Check sheet for the modelled part. Datum: model origin and axes. Units: mm. A direction names the side the tool comes from. Round coordinates to 2 decimals unless told otherwise and drop trailing zeros. Write each loop counter-clockwise with the first axis right and the second up, starting at its lowest first coordinate (ties: lowest second). Pieces come first, ordered by that corner, then holes. Notation, with made-up numbers: (54.5, 56) - (60.5, 56) arc R26 ccw to (60.5, 78) - close; hole circle Ø5 at (84.25, 18). An arc over 180 degrees is marked (long way). Use one line per item in the form item = value. Start each with the question number.
1) Section check A-A (y = 10.5). Record the boundary of the cut face in (x, z) (3 decimals), then the cut area to 3 significant figures.
2) Section check C-C (y = -17.8). Record the boundary of the cut face in (x, z) (3 decimals).
3) Section check B-B (x = 5.75). Record the boundary of the cut face in (y, z) (3 decimals).
4) Section check D-D (x = 11). Record the boundary of the cut face in (y, z).
5) Draft check along X on faces 5 (the face through (-2.93, -17.835, -0.555)), 6 (the face through (3.5, -17.8, -1.6)), 7 (the face through (0, -13.3, -1)), 8 (the face through (12.7, 0, 1)). Enter one of: +X half, -X half, draft (parallel to the pull), parting line (faces both ways), or undercut.
6) Set-up check for faces 1 (the face through (4.301, -16.751, -0.285)), 2 (the face through (-8.2, 16, -1)), 3 (the face through (10.2, 16, -1)), 4 (the face through (8, -18, -2)): record each of +Z, -Z, +X, -X, +Y, -Y from which the full face is reachable in a straight line by a thin tool's end or side.
7) Gauge pin test, flat ends, axial feed: P1, Ø1.6, axis at y = 6.5, z = 3, coming from the +X side (3 decimals); P2, Ø2, axis at x = -9, y = 16, coming from the -Z side; P3, Ø0.5, axis at y = -17.5, z = -1.5, coming from the -X side. Record the tip position at first contact, or that the pin passes through.
8) Scan lines: probe 1 along Y at (x, z) = (0.25, -2); probe 2 along X at (y, z) = (-17, -0.5) (3 decimals); probe 3 along Y at (x, z) = (4, 2) (3 decimals). Record each from-to range of solid material in increasing order.
from build123d import *

# Parameters (mm, degrees)
SKETCH1_W           = 25.4
SKETCH1_H           = 40.6
BOSS_EXTRUDE1_DEPTH = 1.7
SKETCH2_W           = 8
SKETCH2_H           = 7
BOSS_EXTRUDE2_DEPTH = 2.5
CUT_EXTRUDE2_DEPTH  = 5
FILLET1_R           = 1
FILLET2_R           = 1
SKETCH4_W           = 18.8
SKETCH4_H           = 19.2
BOSS_EXTRUDE3_DEPTH = 2.5
SKETCH5_R           = 1.75
BOSS_EXTRUDE4_DEPTH = 2
SKETCH6_W           = 0.5
SKETCH6_H           = 1
BOSS_EXTRUDE5_DEPTH = 0.5
SKETCH7_W           = 2
SKETCH7_H           = 3
BOSS_EXTRUDE6_DEPTH = 2
SKETCH8_W           = 15.875
SKETCH8_H           = 15.875
SKETCH8_H_2         = 19.05
BOSS_EXTRUDE7_DEPTH = 2


with BuildPart() as part:
    # Sketch1 → Boss-Extrude1 (new body)
    with BuildSketch(Plane.XY):
        Rectangle(SKETCH1_W, SKETCH1_H)
    extrude(amount=BOSS_EXTRUDE1_DEPTH)

    # Sketch2 → Boss-Extrude2 (add)
    with BuildSketch(Plane.XY):
        with Locations((0, -16.8)):
            Rectangle(SKETCH2_W, SKETCH2_H)
    extrude(amount=-BOSS_EXTRUDE2_DEPTH)

    # Sketch3 → Cut-Extrude2 (cut)
    with BuildSketch(Plane.XZ.offset(20.3)):
        Polygon((3.5, -2.125), (3.5, -1.125), (2.375, 0), (-2.375, 0), (-3.5, -1.125), (-3.5, -2.125), align=None)
    extrude(amount=-CUT_EXTRUDE2_DEPTH, mode=Mode.SUBTRACT)

    # Fillet1
    fillet1_edges = [part.edges().sort_by_distance(p)[0] for p in [
        (4, -16.8, -2.5),
        (-4, -16.8, -2.5),
    ]]
    fillet(fillet1_edges, radius=FILLET1_R)

    # Fillet2
    fillet2_edges = [part.edges().sort_by_distance(p)[0] for p in [
        (4, -16.8, 0),
        (-4, -16.8, 0),
    ]]
    fillet(fillet2_edges, radius=FILLET2_R)

    # Sketch4 → Boss-Extrude3 (add)
    with BuildSketch(Plane(origin=(0, 0, 0), x_dir=(-1, 0, 0), z_dir=(0, 0, -1))):
        Rectangle(SKETCH4_W, SKETCH4_H)
    extrude(amount=BOSS_EXTRUDE3_DEPTH)

    # Sketch5 → Boss-Extrude4 (add)
    with BuildSketch(Plane(origin=(0, 0, 0), x_dir=(-1, 0, 0), z_dir=(0, 0, -1))):
        with Locations((-8.2, -17.8)):
            Circle(SKETCH5_R)
    extrude(amount=BOSS_EXTRUDE4_DEPTH)

    # Sketch6 → Boss-Extrude5 (add)
    with BuildSketch(Plane(origin=(0, 0, 0), x_dir=(-1, 0, 0), z_dir=(0, 0, -1))):
        with Locations((-7.2, -11.1)):
            Rectangle(SKETCH6_W, SKETCH6_H)
        with Locations((-6.45, -11.1)):
            Rectangle(SKETCH6_W, SKETCH6_H)
    extrude(amount=BOSS_EXTRUDE5_DEPTH)

    # Sketch7 → Boss-Extrude6 (add)
    with BuildSketch(Plane(origin=(0, 0, 0), x_dir=(-1, 0, 0), z_dir=(0, 0, -1))):
        with Locations((-9.2, 16.3)):
            Rectangle(SKETCH7_W, SKETCH7_H)
        with Locations((9.2, 16.3)):
            Rectangle(SKETCH7_W, SKETCH7_H)
    extrude(amount=BOSS_EXTRUDE6_DEPTH)

    # Sketch8 → Boss-Extrude7 (add)
    with BuildSketch(Plane.XY.offset(1.7)):
        with Locations((-1.7625, 9.8625)):
            Rectangle(SKETCH8_W, SKETCH8_H)
        with Locations((0.2375, -9.6)):
            Rectangle(SKETCH8_W, SKETCH8_H_2)
    extrude(amount=BOSS_EXTRUDE7_DEPTH)


solid = part.part
Results are:
q1.outline = (-12.7, 0) - (12.7, 0) - (12.7, 1.7) - (6.175, 1.7) - (6.175, 3.7) - (-9.7, 3.7) - (-9.7, 1.7) - (-12.7, 1.7) - close
q1.area = 74.9 mm²
q2.outline = (-12.7, 0) - (-5, 0) arc R1 cw to (-4, -1) - (-4, -1.5) arc R1 ccw to (-3, -2.5) - (3, -2.5) arc R1 ccw to (4, -1.5) - (4, -1) arc R1 cw to (5, 0) - (6.45, 0) - (6.45, -2) - (9.95, -2) - (9.95, 0) - (12.7, 0) - (12.7, 1.7) - (8.175, 1.7) - (8.175, 3.7) - (-7.7, 3.7) - (-7.7, 1.7) - (-12.7, 1.7) - close; hole (-3.5, -2.125) - (3.5, -2.125) - (3.5, -1.125) - (2.375, 0) - (-2.375, 0) - (-3.5, -1.125) - close
q3.outline = (-20.3, 0) - (-9.6, 0) - (-9.6, -2.5) - (9.6, -2.5) - (9.6, 0) - (20.3, 0) - (20.3, 1.7) - (17.8, 1.7) - (17.8, 3.7) - (1.925, 3.7) - (1.925, 1.7) - (-0.075, 1.7) - (-0.075, 3.7) - (-19.125, 3.7) - (-19.125, 1.7) - (-20.3, 1.7) - close
q4.outline = (-20.3, 0) - (20.3, 0) - (20.3, 1.7) - (-20.3, 1.7) - close
q5.face_5 = undercut
q5.face_6 = undercut
q5.face_7 = draft
q5.face_8 = +X half
q6.face_1 = -Z, -Y
q6.face_2 = -Z, +Y
q6.face_3 = -Z, +X, +Y, -Y
q6.face_4 = -Z, +X, -Y
q7.P1 = 6.175
q7.P2 = -2
q7.P3 = -4
q8.probe_1 = -15.3 to -13.3, -9.6 to 9.6
q8.probe_2 = -4.134 to -2.875, 2.875 to 4.134, 6.644 to 9.756
q8.probe_3 = -19.125 to -0.075, 1.925 to 17.8
